The listing builds one solid part. Answer for the finished solid, in the listing's coordinates (mm). Face numbers are marked on the shaded views. A direction names the side the tool comes from. Round coordinates to 2 decimals unless told otherwise and drop trailing zeros. Write each loop counter-clockwise with the first axis right and the second up, starting at its lowest first coordinate (ties: lowest second). Pieces come first, ordered by that corner, then holes.
Item 1: Find the intervals of material crossed by probe 1 along X at (y, z) = (23.5, 4); probe 2 along Y at (x, z) = (36, -1.5); probe 3 along Z at (x, y) = (32.5, 26), in increasing order.
Item 2: A tool of negligible diameter and unlimited length cuts with its end or side. For the marked faces 1, 2, 3 and 4, from which of +Z, -Z, +X, -X, +Y, -Y can it reach the whole face along a straight path? Write none if from no direction.
Item 3: Find section A-A on z = 7.5. Give the number of separate pieces and of enclosed holes in the cut face, then the cut area to 3 significant figures.
Item 4: Find section B-B on y = 37.5. Give the vertices of the cut face in (x, z).
Item 5: Find section C-C on x = 46. Give the vertices of the cut face in (y, z), then the cut area to 3 significant figures.
Item 6: For a pull along Y with two mould halves and no side action, classify the marked faces 5, 6, 7 and 8 as +Y half, -Y half, draft (parallel to the pull), parting line (faces both ways), or undercut.
Item 7: Find section D-D on z = -7. Give the vertices of the cut face in (x, y).
Item 8: Each of these flat-tipped pins is pushed along its axis until it touches: pin 1 (3 mm diameter, centred on x = 24, z = -2, fed in from -Y); pin 2 (12.5 mm diameter, centred on x = 30.5, y = 32.5, fed in from -Z); pin 3 (4 mm diameter, centred on y = 61.5, z = -11, fed in from -X). Where does it stop, or does it pass through?
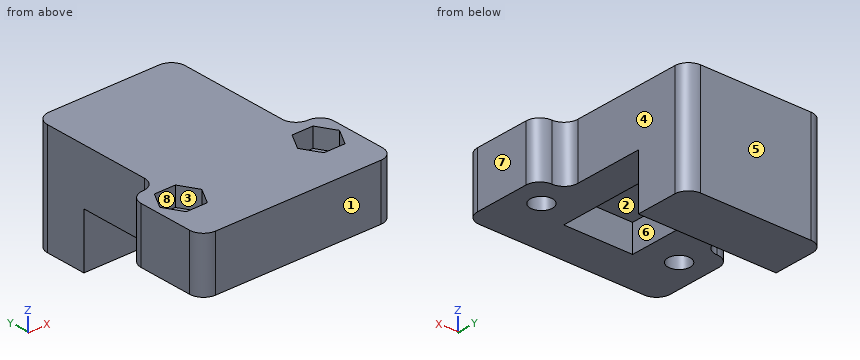
```python
from build123d import *

# Parameters (mm, degrees)
F1_DEPTH  = 20
F3_DEPTH  = 7
F4_R      = 4
F5_DEPTH  = 13.001
F6_R      = 4
F7_DEPTH  = 20.001
F8_W      = 50
F8_H      = 20
F9_DEPTH  = 20
F10_W     = 25
F10_H     = 45
F11_DEPTH = 10
F12_R     = 4.99999


# Not quite as in the source:
# - a fillet or chamfer is up to 0.001 mm smaller than in the source, because OpenCascade refuses the exact size


with BuildPart() as f1:
    # F0 (on Top) → F1 (new body)
    with BuildSketch(Plane.XY):
        Polygon((0, 30), (0, 0), (70, 0), (70, 30), (60, 30), (60, 80), (10, 80), (10, 30), align=None)
    extrude(amount=F1_DEPTH)

    # F2 (on face) → F3 (cut)
    with BuildSketch(Plane.XY.offset(20)):
        Polygon((63.8105117767, 13.4), (67.6210235533, 20), (63.8105117767, 26.6), (56.1894882233, 26.6), (52.3789764467, 20), (56.1894882233, 13.4), align=None)
        Polygon((17.6210235533, 20), (13.8105117767, 26.6), (6.1894882233, 26.6), (2.3789764467, 20), (6.1894882233, 13.4), (13.8105117767, 13.4), align=None)
    extrude(amount=-F3_DEPTH, mode=Mode.SUBTRACT)

    # F4 (on face) → F5 (cut, through all)
    with BuildSketch(Plane.XY.offset(13)):
        with Locations((10, 20)):
            Circle(F4_R)
    extrude(amount=-F5_DEPTH, mode=Mode.SUBTRACT)

    # F6 (on face) → F7 (cut, through all)
    with BuildSketch(Plane.XY.offset(20)):
        with Locations((60, 20)):
            Circle(F6_R)
    extrude(amount=-F7_DEPTH, mode=Mode.SUBTRACT)

    # F8 (on face) → F9 (join)
    with BuildSketch(Plane(origin=(0, 0, 0), x_dir=(1, 0, 0), z_dir=(0, 0, -1))):
        with Locations((35, -70)):
            Rectangle(F8_W, F8_H)
    extrude(amount=F9_DEPTH)

    # F10 (on face) → F11 (cut)
    with BuildSketch(Plane(origin=(0, 0, 0), x_dir=(1, 0, 0), z_dir=(0, 0, -1))):
        with Locations((35, -37.5)):
            Rectangle(F10_W, F10_H)
    extrude(amount=-F11_DEPTH, mode=Mode.SUBTRACT)

    # F12 (radius 5 in the source; OpenCascade refuses exactly that, so slightly less here)
    f12_edges = [f1.edges().sort_by_distance(p)[0] for p in [
        (10, 80, 0),
        (10, 30, 10),
        (60, 30, 10),
        (70, 30, 10),
        (70, 0, 10),
        (0, 0, 10),
        (0, 30, 10),
        (60, 80, 0),
    ]]
    fillet(f12_edges, radius=F12_R)


solid = f1.part
```
Check values:
1. probe 1: x = 0 to 8.06, 11.94 to 22.5, 47.5 to 58.06, 61.94 to 70
1. probe 2: y = 60 to 80
1. probe 3: z = 10 to 20
2. face 1: +Z, -Z, +X, -X, -Y
2. face 2: -Z
2. face 3: +Z
2. face 4: +Z, -Z, +X, +Y
3. separate pieces: 1
3. enclosed holes: 3
3. area: 3,350 mm2
4. outline: (10, 0) - (22.5, 0) - (22.5, 10) - (47.5, 10) - (47.5, 0) - (60, 0) - (60, 20) - (10, 20) - close
5. outline: (0, 0) - (15, 0) - (15, 10) - (60, 10) - (60, -20) - (80, -20) - (80, 20) - (0, 20) - close
5. area: 1,550 mm2
6. face 5: +Y half
6. face 6: undercut
6. face 7: draft
6. face 8: undercut
7. outline: (10, 60) - (60, 60) - (60, 75) arc R5 ccw to (55, 80) - (15, 80) arc R5 ccw to (10, 75) - close
8. pin 1: stops at y = 60
8. pin 2: stops at z = 10
8. pin 3: stops at x = 10
